Check sheet for the modelled part. Datum: model origin and axes. Units: mm. Face numbers are marked on the shaded views. Give positions to 0.01 mm unless a question says otherwise; leave off trailing zeros. Loops run counter-clockwise (first coordinate to the right, second up) from the corner with the lowest first, then second, coordinate; pieces in that order, holes last. Notation, with made-up numbers: (79.5, 46.5) - (117.5, 46.5) arc R25 cw to (117.5, 74.5) - close; hole circle Ø9 at (36.25, -35.5). An arc over 180 degrees is marked (long way). Use CSV: the item, a comma, the result in double quotes.
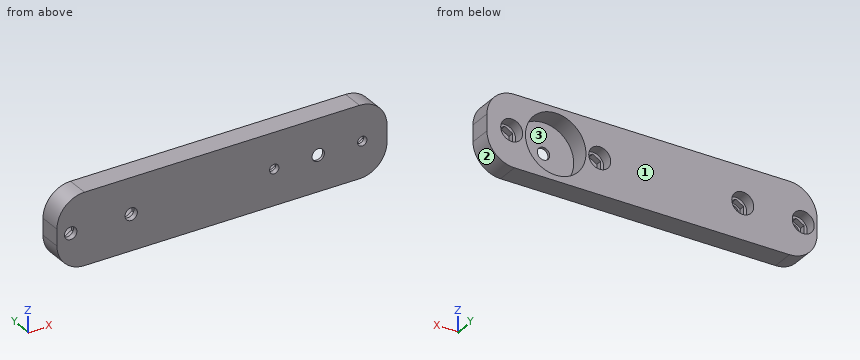
from build123d import *

# Parameters (mm, degrees)
SKETCH1_W                = 120
SKETCH1_H                = 26
BOSS_EXTRUDE1_DEPTH      = 8
SKETCH2_R                = 11
CUT_EXTRUDE1_DEPTH       = 7
SKETCH5_R                = 2.25
CUT_EXTRUDE2_DEPTH       = 2
SKETCH6_R                = 4
CUT_EXTRUDE3_DEPTH       = 4
CUT_EXTRUDE4_DEPTH       = 2.2
M3_CLEARANCE_HOLE1_D     = 3.4
M3_CLEARANCE_HOLE1_DEPTH = 1.8
M4_CLEARANCE_HOLE1_D     = 4.5
SKETCH10_R               = 4
CUT_EXTRUDE5_DEPTH       = 4
CUT_EXTRUDE6_DEPTH       = 2
FILLET1_R                = 10


with BuildPart() as part:
    # Sketch1 → Boss-Extrude1 (new body)
    with BuildSketch(Plane(origin=(0, 0, 0), x_dir=(1, 0, 0), z_dir=(0, 1, 0))):
        Rectangle(SKETCH1_W, SKETCH1_H)
    extrude(amount=BOSS_EXTRUDE1_DEPTH)

    # Sketch2 → Cut-Extrude1 (cut)
    with BuildSketch(Plane(origin=(0, 8, 0), x_dir=(1, 0, 0), z_dir=(0, 1, 0))):
        with Locations((35, 0)):
            Circle(SKETCH2_R)
    extrude(amount=-CUT_EXTRUDE1_DEPTH, mode=Mode.SUBTRACT)

    # Sketch5 → Cut-Extrude2 (cut, through all)
    with BuildSketch(Plane(origin=(0, 1, 0), x_dir=(1, 0, 0), z_dir=(0, 1, 0))):
        with Locations((35, 0)):
            Circle(SKETCH5_R)
    extrude(amount=-CUT_EXTRUDE2_DEPTH, mode=Mode.SUBTRACT)

    # Sketch6 → Cut-Extrude3 (cut)
    with BuildSketch(Plane(origin=(0, 8, 0), x_dir=(1, 0, 0), z_dir=(0, 1, 0))):
        with Locations((51, 0)):
            Circle(SKETCH6_R)
        with Locations((19, 0)):
            Circle(SKETCH6_R)
    extrude(amount=-CUT_EXTRUDE3_DEPTH, mode=Mode.SUBTRACT)

    # Sketch7 → Cut-Extrude4 (cut)
    with BuildSketch(Plane(origin=(0, 4, 0), x_dir=(1, 0, 0), z_dir=(0, 1, 0))):
        Polygon((53.875, -1.659882024), (53.875, 1.659882024), (51, 3.319764048), (48.125, 1.659882024), (48.125, -1.659882024), (51, -3.319764048), align=None)
        Polygon((19, -3.319764048), (16.125, -1.659882024), (16.125, 1.659882024), (19, 3.319764048), (21.875, 1.659882024), (21.875, -1.659882024), align=None)
    extrude(amount=-CUT_EXTRUDE4_DEPTH, mode=Mode.SUBTRACT)

    # M3 Clearance Hole1
    with Locations(Plane(origin=(0, 1.8, 0), x_dir=(1, 0, 0), z_dir=(0, 1, 0))):
        with Locations((51, 0), (19, 0)):
            Hole(M3_CLEARANCE_HOLE1_D / 2, depth=M3_CLEARANCE_HOLE1_DEPTH)

    # M4 Clearance Hole1 (through all)
    with Locations(Plane(origin=(0, 8, 0), x_dir=(1, 0, 0), z_dir=(0, 1, 0))):
        with Locations((-33, 0), (-55, 0)):
            Hole(M4_CLEARANCE_HOLE1_D / 2)

    # Sketch10 → Cut-Extrude5 (cut)
    with BuildSketch(Plane(origin=(0, 8, 0), x_dir=(1, 0, 0), z_dir=(0, 1, 0))):
        with Locations((-55, 0)):
            Circle(SKETCH10_R)
        with Locations((-33, 0)):
            Circle(SKETCH10_R)
    extrude(amount=-CUT_EXTRUDE5_DEPTH, mode=Mode.SUBTRACT)

    # Sketch11 → Cut-Extrude6 (cut)
    with BuildSketch(Plane(origin=(0, 4, 0), x_dir=(1, 0, 0), z_dir=(0, 1, 0))):
        Polygon((-55, -3.319764048), (-52.125, -1.659882024), (-52.125, 1.659882024), (-55, 3.319764048), (-57.875, 1.659882024), (-57.875, -1.659882024), align=None)
        Polygon((-35.875, -1.659882024), (-33, -3.319764048), (-30.125, -1.659882024), (-30.125, 1.659882024), (-33, 3.319764048), (-35.875, 1.659882024), align=None)
    extrude(amount=-CUT_EXTRUDE6_DEPTH, mode=Mode.SUBTRACT)

    # Fillet1
    fillet1_edges = [part.edges().sort_by_distance(p)[0] for p in [
        (-60, 4, -13),
        (60, 4, -13),
        (60, 4, 13),
        (-60, 4, 13),
    ]]
    fillet(fillet1_edges, radius=FILLET1_R)


solid = part.part
1. Scan lines: line 1 along X through (y, z) = (5.75, 0); line 2 along Y through (x, z) = (34, -8); line 3 along Z through (x, y) = (48, 6). Record each from-to range of solid material in increasing order.
Completed:
line 1,"x = -60 to -59, -51 to -37, -29 to 15, 23 to 24, 46 to 47, 55 to 60"
line 2,"y = 0 to 1"
line 3,"z = -13 to -2.65, 2.65 to 13"
2. Sectioned sample at A-A, the plane x = 35. Record the boundary of the cut face in (y, z).
Completed:
outline,"(0, -13) - (8, -13) - (8, -11) - (1, -11) - (1, -2.25) - (0, -2.25) - close; (0, 2.25) - (1, 2.25) - (1, 11) - (8, 11) - (8, 13) - (0, 13) - close"
3. Sectioned sample at B-B, the plane z = 0. State how many separate pieces and enclosed holes the cut face has, and give its area (3 significant figures).
Completed:
separate pieces,"6"
enclosed holes,"0"
area,"595 mm²"
4. Sectioned sample at C-C, the plane z = 10. Record the boundary of the cut face in (x, y).
Completed:
outline,"(-57.14, 0) - (57.14, 0) - (57.14, 8) - (39.58, 8) - (39.58, 1) - (30.42, 1) - (30.42, 8) - (-57.14, 8) - close"
5. Sectioned sample at D-D, the plane z = 5. Record the boundary of the cut face in (x, y).
Completed:
outline,"(-59.8, 0) - (59.8, 0) - (59.8, 8) - (44.8, 8) - (44.8, 1) - (25.2, 1) - (25.2, 8) - (-59.8, 8) - close"
6. Release check for a two-part mould opening along X. For the marked faces 1, 2 and 3 record: released by +X, released by -X, zero draft, split by the parting line, or undercut.
Completed:
face 1,"zero draft"
face 2,"released by +X"
face 3,"undercut"
7. Go/stop test with flat-tipped pins: pin 1 Ø6.5 at (x, z) = (36.5, -0.5) entering from +Y; pin 2 Ø7 at (x, z) = (-33, 0) entering from -Y; pin 3 Ø5 at (x, z) = (-33, 0) entering from +Y; pin 4 Ø2.5 at (x, z) = (-33.5, 0) entering from +Y. Record where each tip stops, or that it passes through.
Completed:
pin 1,"stops at y = 1"
pin 2,"stops at y = 0"
pin 3,"stops at y = 2"
pin 4,"passes through"
